from build123d import *

# Parameters (mm, degrees)
ESQUISSE1_R        = 1.5
BOSS_EXTRU_1_DEPTH = 5


with BuildPart() as part:
    # Esquisse1 → Boss.-Extru.1 (new body)
    with BuildSketch(Plane.XY):
        Polygon((0, 0), (35, 0), (35, 60), (0, 60), (0, 50), (0, 10), align=None)
        with Locations((5, 53.5)):
            Circle(ESQUISSE1_R, mode=Mode.SUBTRACT)
        with Locations(Location((15, 53.5, 0), (0, 0, 180))):
            Circle(ESQUISSE1_R, mode=Mode.SUBTRACT)
        with Locations((15, 6.5)):
            Circle(ESQUISSE1_R, mode=Mode.SUBTRACT)
        with Locations(Location((5, 6.5, 0), (0, 0, 180))):
            Circle(ESQUISSE1_R, mode=Mode.SUBTRACT)
    extrude(amount=BOSS_EXTRU_1_DEPTH)


solid = part.part
Check sheet for the modelled part. Datum: model origin and axes. Units: mm. Round coordinates to 2 decimals unless told otherwise and drop trailing zeros. Write each loop counter-clockwise with the first axis right and the second up, starting at its lowest first coordinate (ties: lowest second). Pieces come first, ordered by that corner, then holes. Notation, with made-up numbers: (-8, 8) - (-3, 8) arc R14 ccw to (-3, 24) - close; hole circle Ø9 at (-25, 37). An arc over 180 degrees is marked (long way). Return JSON: item names as keys, results as strings.
Q1. Scan lines: L1, parallel to Y at x = 15, z = 2.65; L2, parallel to X at y = 54, z = 0.4. Record each from-to range of solid material in increasing order. Write a range as from..to.
Returned:
{"L1": "y = 0..5, 8..52, 55..60", "L2": "x = 0..3.59, 6.41..13.59, 16.41..35"}
Q2. Cross-section at B-B (y = 6.5). Record the boundary of the cut face in (x, z).
Returned:
{"outline": "(0, 0) - (3.5, 0) - (3.5, 5) - (0, 5) - close; (6.5, 0) - (13.5, 0) - (13.5, 5) - (6.5, 5) - close; (16.5, 0) - (35, 0) - (35, 5) - (16.5, 5) - close"}
Q3. Draft check along Y on faces 1 (the cylindrical face through (16.2, 54.4, 2.5)), 2 (the flat face through (18, 60, 2)), 3 (the flat face through (17, 30, 0)), 4 (the cylindrical face through (13.5, 6.57, 2.46)). Enter one of: released by +Y, released by -Y, zero draft, split by the parting line, or undercut.
Returned:
{"face 1": "undercut", "face 2": "released by +Y", "face 3": "zero draft", "face 4": "undercut"}
Q4. Cross-section at A-A (x = 15). Record the boundary of the cut face in (y, z), then the cut area to 3 significant figures.
Returned:
{"outline": "(0, 0) - (5, 0) - (5, 5) - (0, 5) - close; (8, 0) - (52, 0) - (52, 5) - (8, 5) - close; (55, 0) - (60, 0) - (60, 5) - (55, 5) - close", "area": "270 mm²"}
